Input: part model. Units: mm. Frame: model coordinates. Give positions to 0.01 mm unless a question says otherwise; leave off trailing zeros. Order: outer loops, then holes, each group sorted by start corner. A loop starts at its lowest first (then second) coordinate and runs counter-clockwise, first axis right, second up. Notation, with made-up numbers: (7, 55) - (50, 55) arc R15 cw to (50, 76) - close; hole circle Ø10 at (12, -17). An arc over 180 degrees is marked (long way). Use a Markdown table: item, result.
from build123d import *

# Parameters (mm, degrees)
SKETCH1_W                              = 1320.8
SKETCH1_H                              = 12.7
BOSS_EXTRUDE1_DEPTH                    = 2540
SKETCH2_W                              = 660.4
SKETCH2_H                              = 508
CUT_EXTRUDE1_DEPTH                     = 13.7
F_3_8_0_375_DIAMETER_HOLE1_D           = 9.525
F_3_8_0_375_DIAMETER_HOLE1_CSINK_D     = 10.795
F_3_8_0_375_DIAMETER_HOLE1_CSINK_ANGLE = 90
SKETCH5_W                              = 939.8
SKETCH5_H                              = 152.4
CUT_EXTRUDE3_DEPTH                     = 1
CUT_EXTRUDE3_DEPTH_BACK                = 13.7
SKETCH6_R                              = 22.225
CUT_EXTRUDE4_DEPTH                     = 31.75


with BuildPart() as part:
    # Sketch1 → Boss-Extrude1 (new body)
    with BuildSketch(Plane.XY):
        with Locations((660.4, 6.35)):
            Rectangle(SKETCH1_W, SKETCH1_H)
    extrude(amount=BOSS_EXTRUDE1_DEPTH)

    # Sketch2 → Cut-Extrude1 (cut, through all)
    with BuildSketch(Plane(origin=(0, 12.7, 0), x_dir=(1, 0, 0), z_dir=(0, 1, 0))):
        with Locations((660.4, -2286)):
            Rectangle(SKETCH2_W, SKETCH2_H)
    extrude(amount=-CUT_EXTRUDE1_DEPTH, mode=Mode.SUBTRACT)

    # 3/8 (0.375) Diameter Hole1 (through all)
    with Locations(Plane(origin=(0, 12.7, 0), x_dir=(1, 0, 0), z_dir=(0, 1, 0))):
        with Locations((1308.1, -2286), (1308.1, -1828.8), (1308.1, -1371.6), (1308.1, -914.4), (12.7, -2286), (12.7, -1828.8), (12.7, -1371.6), (12.7, -914.4), (495.3, -12.7), (127, -12.7), (1193.8, -12.7), (825.5, -12.7)):
            CounterSinkHole(F_3_8_0_375_DIAMETER_HOLE1_D / 2, F_3_8_0_375_DIAMETER_HOLE1_CSINK_D / 2, counter_sink_angle=F_3_8_0_375_DIAMETER_HOLE1_CSINK_ANGLE)

    # Sketch5 → Cut-Extrude3 (cut, two sides)
    with BuildSketch(Plane(origin=(0, 12.7, 0), x_dir=(1, 0, 0), z_dir=(0, 1, 0))) as cut_extrude3_sk:
        with Locations((647.7, -1552.702)):
            Rectangle(SKETCH5_W, SKETCH5_H)
    extrude(amount=CUT_EXTRUDE3_DEPTH, mode=Mode.SUBTRACT)
    extrude(cut_extrude3_sk.sketch, amount=-CUT_EXTRUDE3_DEPTH_BACK, mode=Mode.SUBTRACT)

    # Sketch6 → Cut-Extrude4 (cut)
    with BuildSketch(Plane(origin=(0, 12.7, 0), x_dir=(1, 0, 0), z_dir=(0, 1, 0))):
        with Locations((442.97784899, -738.973935122)):
            Circle(SKETCH6_R)
    extrude(amount=-CUT_EXTRUDE4_DEPTH, mode=Mode.SUBTRACT)


solid = part.part
1. Section query B-B (x = 745.5). Return loops of the section in (y, z), then the cut area to 3 significant figures.
Response:
| item | result |
|---|---|
| outline | (0, 0) - (12.7, 0) - (12.7, 1476.5) - (0, 1476.5) - close; (0, 1628.9) - (12.7, 1628.9) - (12.7, 2032) - (0, 2032) - close |
| area | 23,900 mm^2 |
2. Material intervals for line 1 along X through (y, z) = (6.25, 1371.6); line 2 along Z through (x, y) = (1308.1, 4.5); line 3 along X through (y, z) = (5.75, 2259.5), sorted ascending.
Response:
| item | result |
|---|---|
| line 1 | x = 0 to 7.94, 17.46 to 1303.34, 1312.86 to 1320.8 |
| line 2 | z = 0 to 909.64, 919.16 to 1366.84, 1376.36 to 1824.04, 1833.56 to 2281.24, 2290.76 to 2540 |
| line 3 | x = 0 to 330.2, 990.6 to 1320.8 |
3. Mould query, pull axis Z, two halves, no side actions, for faces 1 (the face through (651, 0, 970)), 2 (the face through (440.08, 6.44, 716.94)). Classes: pulls with the +Z half, pulls with the -Z half, needs draft (parallel to the pull), parting line crosses it, or undercut.
Response:
| item | result |
|---|---|
| face 1 | needs draft |
| face 2 | undercut |
4. Section query C-C (y = 9.5). State how many separate pieces and enclosed holes the cut face has, then the cut area to 3 significant figures.
Response:
| item | result |
|---|---|
| separate pieces | 1 |
| enclosed holes | 14 |
| area | 2,870,000 mm^2 |
5. Section query A-A (z = 1563). Return loops of the section in (x, y), then the cut area to 3 significant figures.
Response:
| item | result |
|---|---|
| outline | (0, 0) - (177.8, 0) - (177.8, 12.7) - (0, 12.7) - close; (1117.6, 0) - (1320.8, 0) - (1320.8, 12.7) - (1117.6, 12.7) - close |
| area | 4,840 mm^2 |
6. Pin query (flat end, axial travel): pin 1 (2 mm diameter, centred on x = 557.5, y = 2.5, fed in from +Z). Return the tip coordinate at first contact, or that it passes through.
Response:
| item | result |
|---|---|
| pin 1 | stops at z = 2032 |
